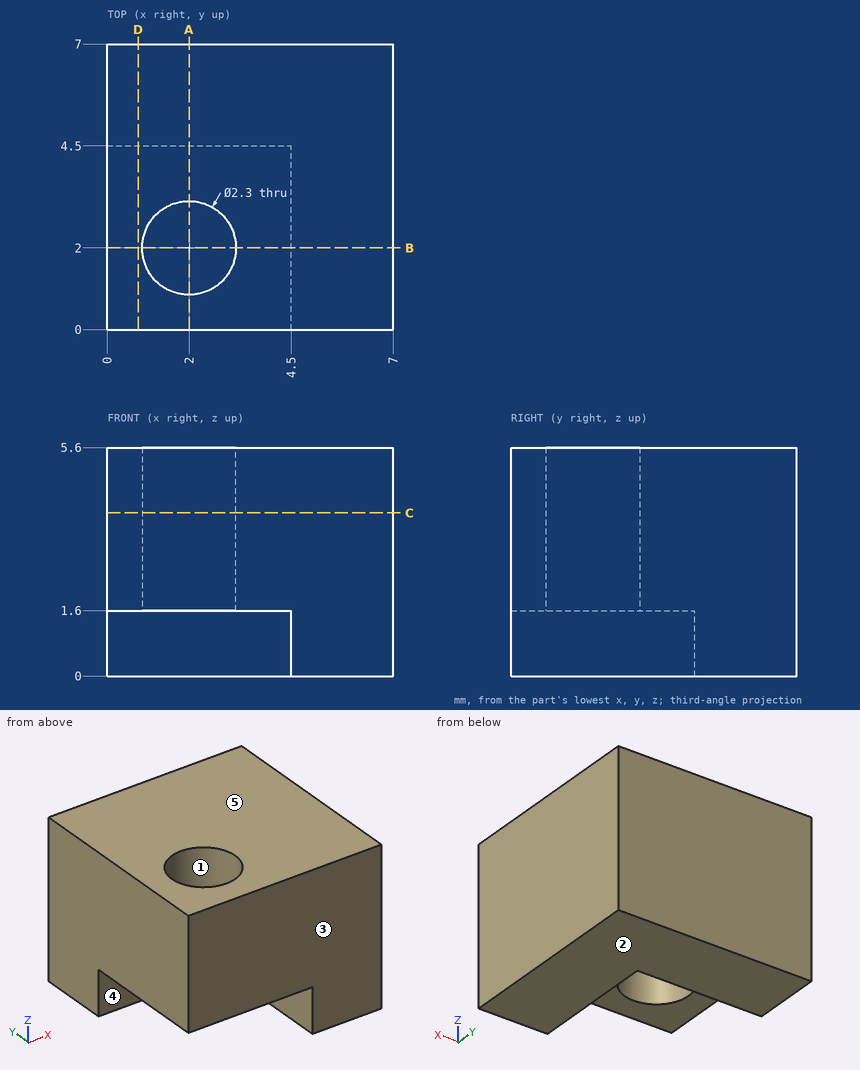
For this review, use the dimensioned drawing (mm, ordinates from the lowest corner) and the shaded views. A direction names the side the tool comes from. Coordinates: 2 decimals unless noted, no trailing zeros. Loops run counter-clockwise (first coordinate to the right, second up) from the corner with the lowest first, then second, coordinate; pieces in that order, holes last. Notation, with made-up numbers: (16.25, 45) -> (74.25, 45) arc R25 cw to (74.25, 83) -> close; hole circle Ø1 at (-17, 60.25). An arc over 180 degrees is marked (long way). Use a Markdown table: item, result. Add a question column.
1. Clearance check with flat-ended pins moving along their axes: pin 1 Ø1.3 at (x, y) = (2.5, 1.5) entering from -Z; pin 2 Ø0.5 at (y, z) = (3, 1) entering from -X; pin 3 Ø1 at (x, z) = (3.5, 4.5) entering from -Y; pin 4 Ø0.5 at (x, z) = (1.5, 0.5) entering from -Y. State where each tip first meets the part, or that it passes through.
2. Add section C-C on z = 4. Write out the cut boundary in (x, y), plus the area to 3 significant figures.
3. Machinability: for the marked faces 4 and 5, which of the approach directions +Z, -Z, +X, -X, +Y, -Y give a long, thin tool a straight path to every point of the face, cutting with its end or side? Answer none if there is none.
4. Draft analysis for pull direction Y (two halves, no side actions). For the marked faces 1, 2 and 3, state which applies: pulls with the +Y half, pulls with the -Y half, needs draft (parallel to the pull), parting line crosses it, or undercut.
5. Add section D-D on x = 0.75. Write out the cut boundary in (y, z).
6. Add section A-A on x = 2. Write out the cut boundary in (y, z).
7. To check wall thickness, follow line 1 (X direction, y = 2, z = 3.55); line 2 (Z direction, x = 3, y = 4). State the ranges of each line that lie inside material, in increasing order.
Returned:
| question | item | result |
|---|---|---|
| 1 | pin 1 | stops at z = 1.6 |
| 1 | pin 2 | stops at x = 4.5 |
| 1 | pin 3 | stops at y = 0 |
| 1 | pin 4 | stops at y = 4.5 |
| 2 | outline | (0, 0) -> (7, 0) -> (7, 7) -> (0, 7) -> close; hole circle Ø2.3 at (2, 2) |
| 2 | area | 44.8 mm² |
| 3 | face 4 | -Z, -X, -Y |
| 3 | face 5 | +Z, +X, -X, +Y, -Y |
| 4 | face 1 | undercut |
| 4 | face 2 | needs draft |
| 4 | face 3 | pulls with the -Y half |
| 5 | outline | (0, 1.6) -> (4.5, 1.6) -> (4.5, 0) -> (7, 0) -> (7, 5.6) -> (0, 5.6) -> close |
| 6 | outline | (0, 1.6) -> (0.85, 1.6) -> (0.85, 5.6) -> (0, 5.6) -> close; (3.15, 1.6) -> (4.5, 1.6) -> (4.5, 0) -> (7, 0) -> (7, 5.6) -> (3.15, 5.6) -> close |
| 7 | line 1 | x = 0 to 0.85, 3.15 to 7 |
| 7 | line 2 | z = 1.6 to 5.6 |
